from build123d import *

# Parameters (mm, degrees)
ESQUISSE1_W             = 15
ESQUISSE1_H             = 7.802319197
BOSS_EXTRU_1_DEPTH      = 10
ESQUISSE2_W             = 55
ESQUISSE2_H             = 12.802319197
ESQUISSE2_W_2           = 40
ESQUISSE2_H_2           = 13
ESQUISSE2_H_3           = 25
BOSS_EXTRU_2_DEPTH      = 10
ESQUISSE3_W             = 60
ESQUISSE3_H             = 12.802319197
BOSS_EXTRU_3_DEPTH      = 10
CONG_1_R                = 10
ESQUISSE4_R             = 1
ENL_V_MAT_EXTRU_1_DEPTH = 276.282402739


with BuildPart() as part:
    # Esquisse1 → Boss.-Extru.1 (new body)
    with BuildSketch(Plane.XY.offset(40)):
        Polygon((-166.141434162, -130.464178298), (-121.141434162, -130.464178298), (-121.141434162, -100.464178298), (-181.141434162, -100.464178298), (-181.141434162, -130.464178298), align=None)
        with Locations((-173.641434162, -134.365337897)):
            Rectangle(ESQUISSE1_W, ESQUISSE1_H)
    extrude(amount=BOSS_EXTRU_1_DEPTH)

    # Esquisse2 → Boss.-Extru.2 (add)
    with BuildSketch(Plane(origin=(0, 0, 40), x_dir=(-1, 0, 0), z_dir=(0, 0, -1))):
        with Locations((208.641434162, -131.865337897)):
            Rectangle(ESQUISSE2_W, ESQUISSE2_H)
        Polygon((181.141434162, -138.266497495), (181.141434162, -125.464178298), (166.141434162, -125.464178298), (166.141434162, -130.464178298), (166.141434162, -138.266497495), align=None)
        Polygon((181.141434162, -100.464178298), (161.141434162, -100.464178298), (161.141434162, -113.464178298), (161.141434162, -125.464178298), (166.141434162, -125.464178298), (181.141434162, -125.464178298), align=None)
        with Locations((141.141434162, -106.964178298)):
            Rectangle(ESQUISSE2_W_2, ESQUISSE2_H_2)
        with Locations((208.641434162, -112.964178298)):
            Rectangle(ESQUISSE2_W, ESQUISSE2_H_3)
    extrude(amount=BOSS_EXTRU_2_DEPTH)

    # Esquisse3 → Boss.-Extru.3 (add)
    with BuildSketch(Plane(origin=(0, 0, 30), x_dir=(-1, 0, 0), z_dir=(0, 0, -1))):
        with Locations((196.141434162, -131.865337897)):
            Rectangle(ESQUISSE3_W, ESQUISSE3_H)
    extrude(amount=BOSS_EXTRU_3_DEPTH)

    # Congé1
    cong_1_edges = [part.edges().sort_by_distance(p)[0] for p in [
        (-121.141434162, -115.464178298, 50),
        (-173.641434162, -138.266497495, 50),
        (-166.141434162, -134.365337896, 50),
        (-143.641434162, -130.464178298, 50),
    ]]
    fillet(cong_1_edges, radius=CONG_1_R - 0.0001)  # a hair under: the kernel refuses the full size

    # Esquisse4 → Enlèv. mat.-Extru.1 (cut, through all)
    with BuildSketch(Plane.XY.offset(50)):
        with Locations((-151.141434162, -123.464178298)):
            Circle(ESQUISSE4_R)
        with Locations((-131.141434162, -123.464178298)):
            Circle(ESQUISSE4_R)
        with Locations((-171.141434162, -128.464178298)):
            Circle(ESQUISSE4_R)
        with Locations((-216.141434162, -128.464178298)):
            Circle(ESQUISSE4_R)
        with Locations(Location((-226.141434162, -110.464178298, 0), (0, 0, 180))):
            Circle(ESQUISSE4_R)
        with Locations(Location((-191.141434162, -110.464178298, 0), (0, 0, 180))):
            Circle(ESQUISSE4_R)
    extrude(amount=-ENL_V_MAT_EXTRU_1_DEPTH, mode=Mode.SUBTRACT)


solid = part.part
Part model, mm, in its own coordinate system. A direction names the side the tool comes from. Give positions to 0.01 mm unless a question says otherwise; leave off trailing zeros. Order: outer loops, then holes, each group sorted by start corner. A loop starts at its lowest first (then second) coordinate and runs counter-clockwise, first axis right, second up. Notation, with made-up numbers: (-22.75, 63) - (1.25, 63) arc R10 cw to (1.25, 70) - close; hole circle Ø5 at (1.5, -32). An arc over 180 degrees is marked (long way). Use a Markdown table: item, result.
1) Saw through at D-D on y = -105. List the corners of the cut face in (x, z), plus the area to 3 significant figures.
Checked values:
| item | result |
|---|---|
| outline | (-236.14, 30) - (-121.14, 30) - (-121.14, 40) arc R10 ccw to (-131.14, 50) - (-181.14, 50) - (-181.14, 40) - (-236.14, 40) - close |
| area | 1,730 mm² |
2) Flat gauge pins, fed straight in: P1, Ø14, axis at y = -131.5, z = 30, coming from the +X side; P2, Ø1.8, axis at x = -131.14, y = -123.46, coming from the -Z side; P3, Ø5, axis at y = -133.5, z = 28, coming from the +X side; P4, Ø5, axis at y = -118.5, z = 43, coming from the +X side. Where does each tip first touch, or does it go through?
Checked values:
| item | result |
|---|---|
| P1 | x = -161.14 |
| P2 | through |
| P3 | x = -166.14 |
| P4 | x = -121.15 |
3) Saw through at B-B on z = 33. List the corners of the cut face in (x, y), plus the area to 3 significant figures.
Checked values:
| item | result |
|---|---|
| outline | (-236.14, -138.27) - (-166.14, -138.27) - (-166.14, -125.46) - (-161.14, -125.46) - (-161.14, -113.46) - (-121.14, -113.46) - (-121.14, -100.46) - (-236.14, -100.46) - close; hole circle Ø2 at (-226.14, -110.46); hole circle Ø2 at (-216.14, -128.46); hole circle Ø2 at (-191.14, -110.46); hole circle Ø2 at (-171.14, -128.46) |
| area | 3,280 mm² |
4) Probe L1, parallel to Z at x = -175.5, y = -127; L2, parallel to Z at x = -159.5, y = -113; L3, parallel to Y at x = -206, z = 24. List the from-to ranges inside material, lowest first. Write a range as from..to.
Checked values:
| item | result |
|---|---|
| L1 | 20..49.98 |
| L2 | 30..50 |
| L3 | -138.27..-125.46 |
5) 3-axis set-ups, long thin cutter, end or side, ignore diameter. For faces 1 (the flat face through (-196, -132, 20)), 2 (the flat face through (-181.141, -119, 45)), 3 (the flat face through (-164, -125.464, 35)), 4 (the cylindrical face through (-148.256, -127.457, 47.148)): which of +Z, -Z, +X, -X, +Y, -Y reach the whole face in a straight line?
Checked values:
| item | result |
|---|---|
| face 1 | -Z, +X, -X, +Y, -Y |
| face 2 | +Z, -X, +Y, -Y |
| face 3 | -Z, +X, -Y |
| face 4 | +Z, +X, -Y |
6) Saw through at C-C on z = 45. List the corners of the cut face in (x, y).
Checked values:
| item | result |
|---|---|
| outline | (-181.14, -136.93) - (-167.48, -136.93) - (-167.48, -129.12) - (-122.48, -129.12) - (-122.48, -100.46) - (-181.14, -100.46) - close; hole circle Ø2 at (-171.14, -128.46); hole circle Ø2 at (-151.14, -123.46); hole circle Ø2 at (-131.14, -123.46) |
